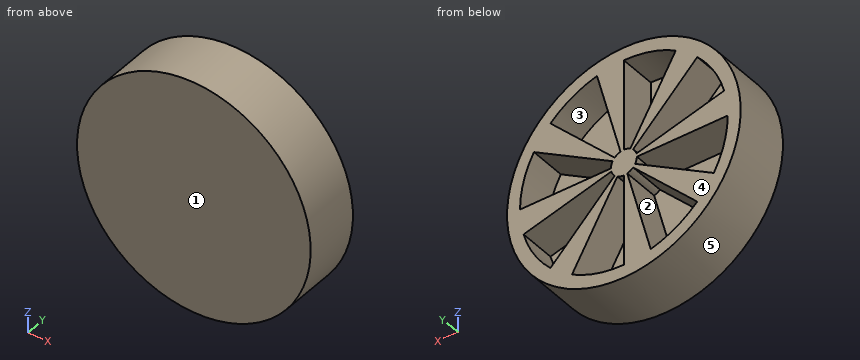
```python
from build123d import *

# Parameters (mm, degrees)
SKETCH1_R                                     = 22.5
MAIN_EXTRUDE_FOR_PLASTIC_MECHANSIM_PART_DEPTH = 11
MAIN_CUT_FOR_PLASTIC_MECHANISM_PART_DEPTH     = 7


with BuildPart() as part:
    # Sketch1 → Main Extrude for Plastic Mechansim Part (new body)
    with BuildSketch(Plane(origin=(0, 0, 0), x_dir=(1, 0, 0), z_dir=(0, 1, 0))):
        with Locations(Location((0, 0, 0), (0, 0, 270))):
            Circle(SKETCH1_R)
    extrude(amount=MAIN_EXTRUDE_FOR_PLASTIC_MECHANSIM_PART_DEPTH)

    # Sketch2 → Main Cut for Plastic Mechanism Part (cut)
    with BuildSketch(Plane(origin=(0, 11, 0), x_dir=(1, 0, 0), z_dir=(0, 1, 0))):
        with BuildLine():
            Line((0, 20), (0, 2.5))
            ThreePointArc((0, 2.5), (0.647047613, 2.414814566), (1.25, 2.165063509))
            Line((1.25, 2.165063509), (10, 17.320508076))
            ThreePointArc((10, 17.320508076), (5.176380902, 19.318516526), (0, 20))
        make_face()
        with BuildLine():
            Line((-20, 0), (-2.5, 0))
            ThreePointArc((-2.5, 0), (-2.414814566, 0.647047613), (-2.165063509, 1.25))
            Line((-2.165063509, 1.25), (-17.320508076, 10))
            ThreePointArc((-17.320508076, 10), (-19.318516526, 5.176380902), (-20, 0))
        make_face()
        with BuildLine():
            Line((-14.142135624, -14.142135624), (-1.767766953, -1.767766953))
            ThreePointArc((-1.767766953, -1.767766953), (-2.165063509, -1.25), (-2.414814566, -0.647047613))
            Line((-2.414814566, -0.647047613), (-19.318516526, -5.176380902))
            ThreePointArc((-19.318516526, -5.176380902), (-17.320508076, -10), (-14.142135624, -14.142135624))
        make_face()
        with BuildLine():
            Line((-14.142135624, 14.142135624), (-1.767766953, 1.767766953))
            ThreePointArc((-1.767766953, 1.767766953), (-1.25, 2.165063509), (-0.647047613, 2.414814566))
            Line((-0.647047613, 2.414814566), (-5.176380902, 19.318516526))
            ThreePointArc((-5.176380902, 19.318516526), (-10, 17.320508076), (-14.142135624, 14.142135624))
        make_face()
        with BuildLine():
            Line((0, -2.5), (0, -20))
            ThreePointArc((0, -20), (-5.176380902, -19.318516526), (-10, -17.320508076))
            Line((-10, -17.320508076), (-1.25, -2.165063509))
            ThreePointArc((-1.25, -2.165063509), (-0.647047613, -2.414814566), (0, -2.5))
        make_face()
        with BuildLine():
            Line((1.767766953, 1.767766953), (14.142135624, 14.142135624))
            ThreePointArc((14.142135624, 14.142135624), (17.320508076, 10), (19.318516526, 5.176380902))
            Line((19.318516526, 5.176380902), (2.414814566, 0.647047613))
            ThreePointArc((2.414814566, 0.647047613), (2.165063509, 1.25), (1.767766953, 1.767766953))
        make_face()
        with BuildLine():
            Line((2.5, 0), (20, 0))
            ThreePointArc((20, 0), (19.318516526, -5.176380902), (17.320508076, -10))
            Line((17.320508076, -10), (2.165063509, -1.25))
            ThreePointArc((2.165063509, -1.25), (2.414814566, -0.647047613), (2.5, 0))
        make_face()
        with BuildLine():
            Line((1.767766953, -1.767766953), (14.142135624, -14.142135624))
            ThreePointArc((14.142135624, -14.142135624), (10, -17.320508076), (5.176380902, -19.318516526))
            Line((5.176380902, -19.318516526), (0.647047613, -2.414814566))
            ThreePointArc((0.647047613, -2.414814566), (1.25, -2.165063509), (1.767766953, -1.767766953))
        make_face()
    extrude(amount=-MAIN_CUT_FOR_PLASTIC_MECHANISM_PART_DEPTH, mode=Mode.SUBTRACT)


solid = part.part
```
Part model, mm, in its own coordinate system. Face numbers are marked on the shaded views. A direction names the side the tool comes from. Round coordinates to 2 decimals unless told otherwise and drop trailing zeros. Write each loop counter-clockwise with the first axis right and the second up, starting at its lowest first coordinate (ties: lowest second). Pieces come first, ordered by that corner, then holes. Notation, with made-up numbers: (12.5, 10.5) -> (57.5, 10.5) arc R19 ccw to (57.5, 15.5) -> close; hole circle Ø2 at (67.25, 28.5). An arc over 180 degrees is marked (long way). Return JSON: item names as keys, results as strings. Group by question number.
Q1. Which spindle directions (+Z, -Z, +X, -X, +Y, -Y) get a long thin tool onto all of the face, cutting with end or side? Do the marked faces 1 and 2. Say none if no direction does.
Q2. Saw through at C-C on z = -13. Write the cut outline in (x, y).
Q3. Probe L1, parallel to Z at x = -5.5, y = 4.5; L2, parallel to X at y = 8.5, z = 12.5; L3, parallel to X at y = 10.25, z = 14. List the from-to ranges inside material, lowest first. Write a range as [from, to].
Q4. Mould opens along Z. For the marked faces 3, 4 and 5 say: pulls with the +Z half, pulls with the -Z half, needs draft (parallel to the pull), parting line crosses it, or undercut.
Q5. Saw through at B-B on x = -6. Write the cut outline in (y, z).
Q6. Saw through at A-A on y = 7.75. State how many separate pieces and enclosed holes the cut face has, plus the area to 3 significant figures.
Q7. Pin check, flat tips, straight feed: pin 1 (4 mm diameter, centred on x = -7, z = -11.5, fed in from +Y); pin 2 (2 mm diameter, centred on y = 2.5, z = 12, fed in from +X); pin 3 (2 mm diameter, centred on y = 7.5, z = 15.5, fed in from -X). Stop position of each tip, or through.
Answer:
{
 "1": {"face 1": "+Z, -Z, +X, -X, -Y", "face 2": "+Y"},
 "2": {"outline": "(-18.36, 0) -> (18.36, 0) -> (18.36, 11) -> (15.2, 11) -> (15.2, 4) -> (13, 4) -> (13, 11) -> (7.51, 11) -> (7.51, 4) -> (0, 4) -> (0, 11) -> (-3.48, 11) -> (-3.48, 4) -> (-13, 4) -> (-13, 11) -> (-18.36, 11) -> close"},
 "3": {"L1": "[-21.82, -19.23], [-5.5, -3.18], [0, 1.47], [5.5, 9.53], [19.23, 21.82]", "L2": "[-18.71, -15.61], [-12.5, -7.22], [0, 3.35], [12.5, 18.71]", "L3": "[-17.61, -14.28], [-14, -8.08], [0, 3.75], [14, 17.61]"},
 "4": {"face 3": "undercut", "face 4": "needs draft", "face 5": "parting line crosses it"},
 "5": {"outline": "(0, -21.69) -> (11, -21.69) -> (11, -19.08) -> (4, -19.08) -> (4, -6) -> (11, -6) -> (11, -3.46) -> (4, -3.46) -> (4, 0) -> (11, 0) -> (11, 1.61) -> (4, 1.61) -> (4, 6) -> (11, 6) -> (11, 10.39) -> (4, 10.39) -> (4, 19.08) -> (11, 19.08) -> (11, 21.69) -> (0, 21.69) -> close"},
 "6": {"separate pieces": "1", "enclosed holes": "8", "area": "766 mm2"},
 "7": {"pin 1": "y = 4", "pin 2": "x = 19.63", "pin 3": "x = -17.2"}
}
